Autodesk Inventor part; units mm, degrees
ref_plane "YZ Plane" through (0, 0, 0) normal (1, 0, 0) x (0, 1, 0)
ref_plane "XZ Plane" through (0, 0, 0) normal (0, 1, 0) x (-1, 0, 0)
ref_plane "XY Plane" through (0, 0, 0) normal (0, 0, 1) x (1, 0, 0)
sketch "Sketch1" plane through (0, 0, 0) normal (0, 1, 0) x (-1, 0, 0)
  circle A0 centre (0, 0) radius 10
  circle A1 centre (0, 0) radius 6.7
  circle A2 centre (0, 0) radius 7.7
  line L0 (-10, 8) -> (-10, -8)
  line L1 (0, 0) -> (-40.0758, 0) construction
  line L2 (-5, 8) -> (-30, 8)
  line L3 (-30, 8) -> (-30, 14)
  line L4 (-30, 14) -> (-5, 14)
  line L5 (-5, 14) -> (-5, 8)
  line L6 (-5, -8) -> (-30, -8)
  line L7 (-30, -8) -> (-30, -14)
  line L8 (-30, -14) -> (-5, -14)
  line L9 (-5, -14) -> (-5, -8)
  line L10 (0, -10) -> (-5, -11)
  line L11 (0, 10) -> (-5, 11)
  point P0 (-10, 0)
  point P1 (-10, 0)
  point P2 (2.5508, 9.6692)
  point P3 (2.5508, -9.6692)
  point P4 (-30, 11)
  point P5 (-10, 8)
  point P6 (-5, 8.6603)
  point P7 (-5, -8.6603)
  point P8 (-6, -8)
  point P9 (-6, 8)
  dimension "d0" = 13.4
  dimension "d1" = 15.4
  dimension "d37" = 20
  dimension "d38" = 20
  dimension "d39" = 6
  dimension "d40" = 5
  dimension "d46" = 16
extrude "Extrusion1" add sketch "Sketch1" along normal blind 2 contours A0 L9 L6 L2 L5 | A0 L5 L11 | L10 L9 A0 | L5 L2 A0 | A0 L2 L3 L4 L5 | L9 L8 L7 L6 A0 | A0 L6 L9 | A0 L0 L2 | L6 L0 A0 | A2
extrude "Extrusion2" add sketch "Sketch1" against normal blind 30 contours A0 L9 L6 L2 L5 | A0 L5 L11 | L10 L9 A0 | L5 L2 A0 | A0 L2 L3 L4 L5 | L9 L8 L7 L6 A0 | A0 L6 L9 | A0 L0 L2 | L6 L0 A0
sketch "Sketch2" plane through (0, 0, 0) normal (1, 0, 0) x (0, 1, 0)
  circle A0 centre (-25, 0) radius 1.75
  line L0 (-30, -7.7) -> (-30, 7.7)
  point P0 (0, 0)
  dimension "d7" = 3.5
  dimension "d8" = 5
extrude "Extrusion3" cut sketch "Sketch2" along normal mid plane 62.5
fillet "Fillet2" radius 7.5 2 edges at (10, -14, -8) (10, -14, 8)
sketch "Sketch4" plane through (29.508, -30, 14) normal (0, 0, 1) x (1, 0, 0)
  circle A0 centre (-4.508, 6) radius 2.25
  circle A1 centre (-4.508, 16) radius 2.25
  circle A2 centre (-4.508, 26) radius 2.25
  line L0 (-4.508, 6) -> (-4.508, 16) construction
  line L1 (-4.508, 16) -> (-4.508, 26) construction
  line L2 (0.492, 0) -> (0.492, 32)
  point P0 (-29.508, 30)
  point P1 (0.492, 16)
  point P2 (0.492, 16)
  dimension "d32" = 4.5
  dimension "d33" = 10
  dimension "d41" = 5
extrude "Extrusion7" cut sketch "Sketch4" against normal up to surface (28 mm away)
fillet "Fillet5" radius 10 2 edges at (5, -14, -11) (5, -14, 11)
fillet "Fillet6" radius 10 2 edges at (5, -14, -14) (5, -14, 14)
fillet "Fillet7" radius 10 2 edges at (0, -14, 10) (0, -14, -10)
fillet "Fillet4" radius 2 4 edges at (30, -14, -14) (30, -14, -8) (30, -14, 8) (30, -14, 14)
properties part number "button bottom part 1"
Could you check a few things on this model? Use its own coordinates, in mm. A direction names the side the tool comes from. Coordinates: 2 decimals unless noted, no trailing zeros. Write each loop counter-clockwise with the first axis right and the second up, starting at its lowest first coordinate (ties: lowest second). Pieces come first, ordered by that corner, then holes. Notation, with made-up numbers: (-4, -31.5) - (29, -31.5) arc R17 ccw to (29, -19.5) - close; hole circle Ø6 at (-13.75, 5.25). An arc over 180 degrees is marked (long way). Use a Markdown table: item, result.
Q1. Please list where these lines run through material, in increasing order: L1, parallel to Y at x = 25, z = -9.95; L2, parallel to Z at x = 28, y = -4; L3, parallel to Z at x = -2, y = -14.5.
Geometry check:
| item | result |
|---|---|
| L1 | y = -30 to -26.25, -21.75 to -16.25, -11.75 to -6.25, -1.75 to 2 |
| L2 | z = -14 to -8, 8 to 14 |
| L3 | z = -9.8 to -7.44, 7.44 to 9.8 |
Q2. Imagine slicing it at D-D (z = -3). List the corners of the cut face in (x, y) for me.
Geometry check:
| item | result |
|---|---|
| outline | (-9.54, -30) - (-7.09, -30) - (-7.09, 0) - (-5.99, 0) - (-5.99, 2) - (-9.54, 2) - close; (5.99, 0) - (7.09, 0) - (7.09, -30) - (10.43, -30) - (10.43, 2) - (5.99, 2) - close |
Q3. Thinking about a two-plate mould opening in X: for faces 1 (the cylindrical face through (-7.113, -14.79, -2.949)), 2 (the cylindrical face through (12.139, -14.224, -5.745)), 3 (the flat face through (22, -14, -8)), which applies, +X half, -X half, draft (parallel to the pull), parting line (faces both ways), or undercut?
Geometry check:
| item | result |
|---|---|
| face 1 | undercut |
| face 2 | +X half |
| face 3 | draft |
Q4. Imagine slicing it at A-A (x = 18.5). List the corners of the cut face in (y, z) for me.
Geometry check:
| item | result |
|---|---|
| outline | (-30, -14) - (2, -14) - (2, -8) - (-30, -8) - close; (-30, 8) - (2, 8) - (2, 14) - (-30, 14) - close |
Q5. Imagine slicing it at B-B (x = 25). Count the separate pieces of the cut face and the enclosed holes in it, and give its area (3 significant figures).
Geometry check:
| item | result |
|---|---|
| separate pieces | 8 |
| enclosed holes | 0 |
| area | 222 mm2 |
Q6. Which directions (+Z, -Z, +X, -X, +Y, -Y) give clear straight access to the entire face, cutting with the end or side of a thin tool? Please do faces 4 (the cylindrical face through (29.4, -13.78, -8.57)), 5 (the flat face through (19, -14, -14)).
Geometry check:
| item | result |
|---|---|
| face 4 | +X, +Y, -Y |
| face 5 | -Z, +X, -X, +Y, -Y |
Q7. I'm going to push flat-ended pins straight in: pin 1 Ø1 at (x, y) = (-2, -9) entering from +Z; pin 2 Ø4 at (y, z) = (-21, -6) entering from -X; pin 3 Ø4 at (x, y) = (25, -14) entering from +Z; pin 4 Ø2 at (y, z) = (-14, -7.5) entering from +X. Where does each tip first touch, or does it pass through?
Geometry check:
| item | result |
|---|---|
| pin 1 | stops at z = 9.89 |
| pin 2 | stops at x = -9.17 |
| pin 3 | passes through |
| pin 4 | stops at x = 29.32 |
